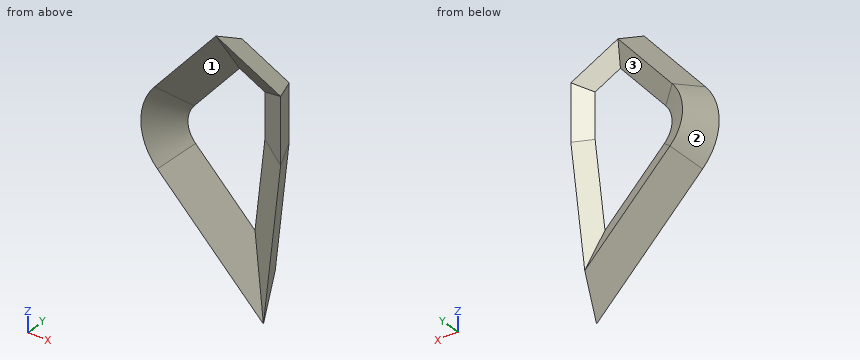
```python
from build123d import *


with BuildPart() as f2:
    # F2: sweep along a path in F1
    with BuildLine(Plane.XZ) as f2_path:
        Line((0, 0), (0, 50.7971271873))
        Line((0, 50.7971271873), (-43.1399196386, 72.9165449739))
        Line((-43.1399196386, 72.9165449739), (-90.9753785277, 16.1548483209))
        ThreePointArc((-90.9753785277, 16.1548483209), (-100.3607226238, -11.1131320772), (-88.9698324182, -37.6060567764))
        Line((-88.9698324182, -37.6060567764), (-12.4816746493, -115.7265843466))
        Line((-12.4816746493, -115.7265843466), (0, 0))
    # F0 (on Top) → F2 (sweep)
    with BuildSketch(Plane.XY):
        Polygon((10.2172587067, -6.4580785111), (-1.9277846441, 20.1453492045), (-16.9645044953, 12.0486542583), align=None)
    sweep(path=f2_path.line, transition=Transition.RIGHT)


solid = f2.part
```
Check sheet for the modelled part. Datum: model origin and axes. Units: mm. Face numbers are marked on the shaded views. A direction names the side the tool comes from. Give positions to 0.01 mm unless a question says otherwise; leave off trailing zeros. Write each loop counter-clockwise with the first axis right and the second up, starting at its lowest first coordinate (ties: lowest second). Pieces come first, ordered by that corner, then holes.
Item 1: Gauge pin test, flat ends, axial feed: pin 1 (2 mm diameter, centred on x = -11, y = 0, fed in from -Z); pin 2 (12 mm diameter, centred on y = -1, z = 32.5, fed in from +X); pin 3 (8 mm diameter, centred on x = -76.5, y = -3, fed in from -Z). Record the tip position at first contact, or that the pin passes through.
Item 2: Cross-section at B-B (z = 42.5). Enter the section's corners in (x, y).
Item 3: Cross-section at A-A (y = -1.25). Enter the section's corners in (x, z).
Item 4: Cross-section at C-C (x = -35.5). Enter the section's corners in (y, z), and give its area (3 significant figures).
Item 5: Access from +Z, -Z, +X, -X, +Y, -Y to the whole of each face (thin tool, end or side, straight path). Record for the marked faces 1, 2 and 3.
Item 6: Cross-section at D-D (z = -103.5). Enter the section's corners in (x, y).
Item 7: Scan lines: L1, parallel to X at y = 4.25, z = 41; L2, parallel to X at y = -2.75, z = -16.5; L3, parallel to Z at x = -95.5, y = -2.5. Record each from-to range of solid material in increasing order.
Report:
1. pin 1: stops at z = -128.84
1. pin 2: stops at x = 10.22
1. pin 3: stops at z = -67.54
2. outline: (-82.13, -6.46) - (-46.59, 12.05) - (-66.25, 20.15) - close; (-21, 12.05) - (-13.58, 9.74) - (10.22, -6.46) - (-1.93, 20.15) - (-13.58, 13.87) - close
3. outline: (-96.97, 21.21) arc R47.84 ccw to (-94.57, -43.09) - (-6.47, -133.07) - (7.84, -0.42) - (7.84, 55.59) - (-45.11, 82.74) - close; hole (-92.94, 17.81) arc R42.57 ccw to (-90.8, -39.4) - (-10.51, -121.41) - (2.57, -0.14) - (2.57, 52.37) - (-43.79, 76.13) - close
4. outline: (-6.46, -106.82) - (20.15, -89.46) - (12.05, -67.97) - close; (-6.46, 80.48) - (12.05, 49.93) - (20.15, 66.83) - close
4. area: 636 mm2
5. face 1: -Y
5. face 2: -X, +Y
5. face 3: +Y
6. outline: (-38.75, -6.46) - (-16.72, 4.26) - (-0.89, -6.46) - (-13.1, 20.15) - (-16.72, 18.21) - (-21.75, 20.15) - close
7. L1: x = -77.01 to -62.83, -5.51 to 5.33
7. L2: x = -108.42 to -104.63, 3.02 to 6.79
7. L3: z = -42.95 to -36.8, 17.56 to 23.84
